Verification items for the finished model (mm, model axes). Round coordinates to 2 decimals unless told otherwise and drop trailing zeros. Write each loop counter-clockwise with the first axis right and the second up, starting at its lowest first coordinate (ties: lowest second). Pieces come first, ordered by that corner, then holes. Notation, with made-up numbers: (48.5, -8) - (72.5, -8) arc R27 ccw to (72.5, 23) - close; hole circle Ø11 at (72, 8). An arc over 180 degrees is marked (long way). Answer as a JSON object with one key per item and string values.
```python
from build123d import *

# Parameters (mm, degrees)
SKETCH1_W           = 125
SKETCH1_H           = 88
BOSS_EXTRUDE1_DEPTH = 3


with BuildPart() as part:
    # Sketch1 → Boss-Extrude1 (new body)
    with BuildSketch(Plane.XY):
        Polygon((60, 128), (60, 131), (30, 131), (30, 128), (0, 128), (0, 104.8), (3, 104.8), (3, 78.6), (0, 78.6), (0, 52.4), (3, 52.4), (3, 26.2), (0, 26.2), (0, 3), (30, 3), (30, 0), (60, 0), (60, 3), (90, 3), (90, 0), (120, 0), (120, 3), (150, 3), (150, 0), (190, 0), (190, 26.2), (187, 26.2), (187, 52.4), (190, 52.4), (190, 78.6), (187, 78.6), (187, 104.8), (190, 104.8), (190, 131), (150, 131), (150, 128), (120, 128), (120, 131), (90, 131), (90, 128), align=None)
        with Locations((69, 62)):
            Rectangle(SKETCH1_W, SKETCH1_H, mode=Mode.SUBTRACT)
    extrude(amount=BOSS_EXTRUDE1_DEPTH)


solid = part.part
```
Q1. Section check A-A, the plane x = 100.5. Record the cut outline in (y, z), then the cut area to 3 significant figures.
Geometry check:
{"outline": "(0, 0) - (18, 0) - (18, 3) - (0, 3) - close; (106, 0) - (131, 0) - (131, 3) - (106, 3) - close", "area": "129 mm2"}
Q2. Material ranges on line 1 along Y through (x, z) = (122, 0.9); line 2 along Y through (x, z) = (52, 0.9); line 3 along X through (y, z) = (40, 1.6), recorded low to high. Write a range as [from, to].
Geometry check:
{"line 1": "y = [3, 18], [106, 128]", "line 2": "y = [0, 18], [106, 131]", "line 3": "x = [3, 6.5], [131.5, 187]"}
Q3. Section check C-C, the plane x = 145.5. Record the cut outline in (y, z), then the cut area to 3 significant figures.
Geometry check:
{"outline": "(3, 0) - (128, 0) - (128, 3) - (3, 3) - close", "area": "375 mm2"}
Q4. Gauge pin test, flat ends, axial feed: P1, Ø1.5, axis at y = 130, z = 2, coming from the -X side; P2, Ø0.9, axis at x = 2, z = 1, coming from the -Y side. Record the tip position at first contact, or that the pin passes through.
Geometry check:
{"P1": "stops at x = 30", "P2": "stops at y = 3"}
Q5. Section check B-B, the plane y = 28.5. Record the cut outline in (x, z), then the cut area to 3 significant figures.
Geometry check:
{"outline": "(3, 0) - (6.5, 0) - (6.5, 3) - (3, 3) - close; (131.5, 0) - (187, 0) - (187, 3) - (131.5, 3) - close", "area": "177 mm2"}
